Read the model definition and answer for the solid it produces. Units are mm, in the model's axes. Face numbers are marked on the shaded views. Give positions to 0.01 mm unless a question says otherwise; leave off trailing zeros. Order: outer loops, then holes, each group sorted by start corner. A loop starts at its lowest first (then second) coordinate and runs counter-clockwise, first axis right, second up.
Item 1: Given pin 1 Ø5 at (x, y) = (-7.5, -20) entering from +Z (3 decimals); pin 2 Ø23.5 at (x, y) = (0, 0) entering from -Z; pin 3 Ø0.6 at (x, z) = (-6, 0.5) entering from -Y, each flat-ended and moving along its own axis, determine where each tip first touches the part or whether it passes through.
Item 2: A cutting plane is placed at C-C (z = 1.55). Write down the section's boundary in (x, y), plus the area to 3 significant figures.
Item 3: A cutting plane is placed at B-B (y = -25.5). Write down the section's boundary in (x, z) (3 decimals).
Item 4: The mould has two halves that part along X. Classify the marked faces 1 and 2: +X half, -X half, draft (parallel to the pull), parting line (faces both ways), or undercut.
Item 5: A cutting plane is placed at A-A (x = 0). Write down the section's boundary in (y, z) (3 decimals).
Item 6: A cutting plane is placed at D-D (x = 29.5). Write down the section's boundary in (y, z) (3 decimals), plus the area to 3 significant figures.
Item 7: Find the intervals of material crossed by line 1 along X through (y, z) = (0, 0.7) (3 decimals); line 2 along Y through (x, z) = (0, 1.5); line 3 along X through (y, z) = (-32, 1.4), in increasing order.
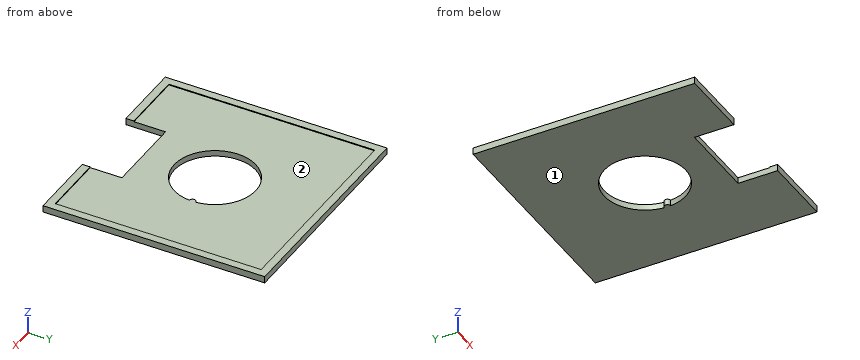
from build123d import *

# Parameters (mm, degrees)
F0_W     = 66.04
F0_H     = 66.04
F1_DEPTH = 1.905
F0_W_2   = 71.12
F0_H_2   = 71.12
F2_DEPTH = 2.159
F3_W     = 25.4
F3_H     = 25.4
F4_DEPTH = 25.4


with BuildPart() as f1:
    # F0 (on Top) → F1 (new body)
    with BuildSketch(Plane.XY):
        Rectangle(F0_W, F0_H)
        with BuildLine():
            ThreePointArc((13.041544, -1.015234), (-13.081, 0), (13.041544, 1.015234))
            ThreePointArc((13.041544, 1.015234), (12.065, 0), (13.041544, -1.015234))
        make_face(mode=Mode.SUBTRACT)
    extrude(amount=F1_DEPTH)

    # F0 (on Top) → F2 (join)
    with BuildSketch(Plane.XY):
        Rectangle(F0_W_2, F0_H_2)
        Rectangle(F0_W, F0_H, mode=Mode.SUBTRACT)
    extrude(amount=F2_DEPTH)

    # F3 (on face) → F4 (cut)
    with BuildSketch(Plane(origin=(0, 0, 0), x_dir=(1, 0, 0), z_dir=(0, 0, -1))):
        with Locations((0, 35.56)):
            Rectangle(F3_W, F3_H)
    extrude(amount=-F4_DEPTH, mode=Mode.SUBTRACT)


solid = f1.part
Response values:
1. pin 1: stops at z = 1.905
1. pin 2: passes through
1. pin 3: stops at y = -22.86
2. outline: (-35.56, -35.56) - (-12.7, -35.56) - (-12.7, -22.86) - (12.7, -22.86) - (12.7, -35.56) - (35.56, -35.56) - (35.56, 35.56) - (-35.56, 35.56) - close; hole (13.04, -1.02) arc R1.02 cw to (13.04, 1.02) arc R13.08 ccw (long way) to start
2. area: 4,200 mm2
3. outline: (-35.56, 0) - (-12.7, 0) - (-12.7, 1.905) - (-33.02, 1.905) - (-33.02, 2.159) - (-35.56, 2.159) - close; (12.7, 0) - (35.56, 0) - (35.56, 2.159) - (33.02, 2.159) - (33.02, 1.905) - (12.7, 1.905) - close
4. face 1: draft
4. face 2: undercut
5. outline: (-22.86, 0) - (-13.081, 0) - (-13.081, 1.905) - (-22.86, 1.905) - close; (13.081, 0) - (35.56, 0) - (35.56, 2.159) - (33.02, 2.159) - (33.02, 1.905) - (13.081, 1.905) - close
6. outline: (-35.56, 0) - (35.56, 0) - (35.56, 2.159) - (33.02, 2.159) - (33.02, 1.905) - (-33.02, 1.905) - (-33.02, 2.159) - (-35.56, 2.159) - close
6. area: 137 mm2
7. line 1: x = -35.56 to -13.081, 12.065 to 35.56
7. line 2: y = -22.86 to -13.08, 13.08 to 35.56
7. line 3: x = -35.56 to -12.7, 12.7 to 35.56
